from build123d import *

# Parameters (mm, degrees)
SKETCH1_W           = 150
SKETCH1_H           = 63.315
BOSS_EXTRUDE1_DEPTH = 6.5
SKETCH2_W           = 4
SKETCH2_H           = 6.5
BOSS_EXTRUDE2_DEPTH = 19
SKETCH3_W           = 30
SKETCH3_H           = 6.5
CUT_EXTRUDE1_DEPTH  = 18.75
CHAMFER1_SIZE       = 5
SKETCH5_R           = 5
BOSS_EXTRUDE3_DEPTH = 17.5
FILLET1_R           = 5
SKETCH6_R           = 3.5
CUT_EXTRUDE2_DEPTH  = 17.5
SKETCH7_R           = 3.5
CUT_EXTRUDE3_DEPTH  = 17.5
SKETCH8_R           = 2
CUT_EXTRUDE4_DEPTH  = 6.5
SKETCH9_R           = 1.5
CUT_EXTRUDE5_DEPTH  = 25


with BuildPart() as part:
    # Sketch1 → Boss-Extrude1 (new body)
    with BuildSketch(Plane(origin=(0, 0, 0), x_dir=(1, 0, 0), z_dir=(0, 1, 0))):
        Rectangle(SKETCH1_W, SKETCH1_H)
    extrude(amount=BOSS_EXTRUDE1_DEPTH)

    # Sketch2 → Boss-Extrude2 (add)
    with BuildSketch(Plane.XY.offset(31.6575)):
        with Locations((-10.5, 3.25)):
            Rectangle(SKETCH2_W, SKETCH2_H)
        with Locations((10.5, 3.25)):
            Rectangle(SKETCH2_W, SKETCH2_H)
    extrude(amount=BOSS_EXTRUDE2_DEPTH)

    # Sketch3 → Cut-Extrude1 (cut)
    with BuildSketch(Plane(origin=(0, 0, -31.6575), x_dir=(-1, 0, 0), z_dir=(0, 0, -1))):
        with Locations((-60, 3.25)):
            Rectangle(SKETCH3_W, SKETCH3_H)
        with Locations((60, 3.25)):
            Rectangle(SKETCH3_W, SKETCH3_H)
    extrude(amount=-CUT_EXTRUDE1_DEPTH, mode=Mode.SUBTRACT)

    # Chamfer1
    chamfer1_edges = [part.edges().sort_by_distance(p)[0] for p in [
        (75, 3.25, -12.9075),
        (45, 3.25, -31.6575),
        (-75, 3.25, -12.9075),
        (-45, 3.25, -31.6575),
    ]]
    chamfer(chamfer1_edges, length=CHAMFER1_SIZE)

    # Sketch5 → Boss-Extrude3 (add)
    with BuildSketch(Plane.XZ):
        with Locations(Location((45, 4.4725, 0), (0, 0, 90))):
            Circle(SKETCH5_R)
        with Locations(Location((-45, 4.4725, 0), (0, 0, 90))):
            Circle(SKETCH5_R)
    extrude(amount=BOSS_EXTRUDE3_DEPTH)

    # Fillet1
    fillet1_edges = [part.edges().sort_by_distance(p)[0] for p in [
        (-45, 0, -0.5275),
        (45, 0, -0.5275),
    ]]
    fillet(fillet1_edges, radius=FILLET1_R)

    # Sketch6 → Cut-Extrude2 (cut)
    with BuildSketch(Plane.XZ.offset(17.5)):
        with Locations(Location((45, 4.4725, 0), (0, 0, 270))):
            Circle(SKETCH6_R)
    extrude(amount=-CUT_EXTRUDE2_DEPTH, mode=Mode.SUBTRACT)

    # Sketch7 → Cut-Extrude3 (cut)
    with BuildSketch(Plane.XZ.offset(17.5)):
        with Locations(Location((-45, 4.4725, 0), (0, 0, 270))):
            Circle(SKETCH7_R)
    extrude(amount=-CUT_EXTRUDE3_DEPTH, mode=Mode.SUBTRACT)

    # Sketch8 → Cut-Extrude4 (cut)
    with BuildSketch(Plane.XZ):
        with Locations(Location((45, 4.4725, 0), (0, 0, 270))):
            Circle(SKETCH8_R)
        with Locations(Location((-45, 4.4725, 0), (0, 0, 270))):
            Circle(SKETCH8_R)
    extrude(amount=-CUT_EXTRUDE4_DEPTH, mode=Mode.SUBTRACT)

    # Sketch9 → Cut-Extrude5 (cut)
    with BuildSketch(Plane.ZY.offset(12.5)):
        with Locations((41.1575, 3.25)):
            Circle(SKETCH9_R)
    extrude(amount=-CUT_EXTRUDE5_DEPTH, mode=Mode.SUBTRACT)


solid = part.part
Work out the finished part from the listing and answer in its coordinate system (mm). A direction names the side the tool comes from. Coordinates: 2 decimals unless noted, no trailing zeros. Write each loop counter-clockwise with the first axis right and the second up, starting at its lowest first coordinate (ties: lowest second). Pieces come first, ordered by that corner, then holes. Notation, with made-up numbers: M 66.25,89.25 L 78.25,89.25 A25 cw 78.25,118.25 Z; hole C 19,10.25 d6. An arc over 180 degrees is marked long. Write item = value, one per line.
1. Determine the mould class of faces 1 (the face through (-1, 3, -31.658)), 2 (the face through (10, 3, 50.658)), 3 (the face through (43.05, 3.2, 4.91)), 4 (the face through (43, 0, 3)) for opening direction Z: released by +Z, released by -Z, zero draft, split by the parting line, or undercut.
Solution:
face_1 = released by -Z
face_2 = released by +Z
face_3 = undercut
face_4 = undercut
2. The part is cut by section B-B (y = -9). Determine the outline of the cut face in (x, z), then the cut area to 3 significant figures.
Solution:
outline = C -45,4.47 d10; C 45,4.47 d10; hole C -45,4.47 d7; hole C 45,4.47 d7
area = 80.1 mm2
3. The part is cut by section C-C (x = -7). Determine the outline of the cut face in (y, z), then the cut area to 3 significant figures.
Solution:
outline = M 0,-31.66 L 6.5,-31.66 L 6.5,31.66 L 0,31.66 Z
area = 412 mm2
4. The part is cut by section A-A (y = 3.25). State how many separate pieces and enclosed holes the cut face has, then the cut area to 3 significant figures.
Solution:
separate_pieces = 3
enclosed_holes = 2
area = 8,430 mm2
5. The part is cut by section D-D (z = -18). Determine the outline of the cut face in (x, y), then the cut area to 3 significant figures.
Solution:
outline = M -45,0 L 45,0 L 45,6.5 L -45,6.5 Z
area = 585 mm2
6. Flat-ended cylindrical pins translate along their axes: pin 1 (5 mm diameter, centred on y = 2.5, z = -21.5, fed in from -X); pin 2 (10 mm diameter, centred on x = 54.5, y = -2, fed in from -Z); pin 3 (5 mm diameter, centred on x = 45, z = 4.47, fed in from +Y); pin 4 (7 mm diameter, centred on y = 5, z = 39, fed in from +X). Find the tip coordinate at first contact, or state that the pin passes through.
Solution:
pin_1 = -45
pin_2 = -12.91
pin_3 = 6.5
pin_4 = 12.5
7. Straight lines are drawn through the part: line 1 (X direction, y = -9.75, z = 4); line 2 (Z direction, x = 61, y = 3.75); line 3 (Y direction, x = 59, z = 15). For each, find the intervals that lie inside material, in ascending order. Write a range as from..to.
Solution:
line_1 = -49.98..-48.47, -41.53..-40.02, 40.02..41.53, 48.47..49.98
line_2 = -12.91..31.66
line_3 = 0..6.5
8. For faces 5 (the face through (-49.957, -11.162, 3.822)), 6 (the face through (58, 3, -12.907)), 7 (the face through (-57, 3, -12.907)), 8 (the face through (-12.5, 3, 39)), determine the directions among +Z, -Z, +X, -X, +Y, -Y from which every point of the face is accessible in a straight line to the end or side of a thin tool.
Solution:
face_5 = -Y
face_6 = -Z, +X, +Y, -Y
face_7 = -Z, -X, +Y, -Y
face_8 = +Z, -X, +Y, -Y
